from build123d import *

# Parameters (mm, degrees)
SKETCH1_W           = 72.771
SKETCH1_H           = 66.9925
SKETCH1_R           = 19.1135
SKETCH1_R_2         = 3.175
BOSS_EXTRUDE1_DEPTH = 3.175
FILLET1_R           = 2.54
SKETCH2_W           = 66.9925
SKETCH2_H           = 50.8
BOSS_EXTRUDE2_DEPTH = 3.175
BOSS_EXTRUDE5_DEPTH = 3.175
BOSS_EXTRUDE6_DEPTH = 3.175
SKETCH9_R           = 3.175
CUT_EXTRUDE1_DEPTH  = 3.175
BOSS_EXTRUDE7_DEPTH = 5.08


with BuildPart() as part:
    # Sketch1 → Boss-Extrude1 (new body)
    with BuildSketch(Plane(origin=(0, 0, 0), x_dir=(1, 0, 0), z_dir=(0, 1, 0))):
        with Locations((-3.302, 0.79375)):
            Rectangle(SKETCH1_W, SKETCH1_H)
        with Locations(Location((0, 0, 0), (0, 0, 270))):
            Circle(SKETCH1_R, mode=Mode.SUBTRACT)
        with Locations(Location((-23.5585, 23.5585, 0), (0, 0, 270))):
            Circle(SKETCH1_R_2, mode=Mode.SUBTRACT)
        with Locations(Location((23.5585, 23.5585, 0), (0, 0, 270))):
            Circle(SKETCH1_R_2, mode=Mode.SUBTRACT)
        with Locations(Location((23.5585, -23.5585, 0), (0, 0, 270))):
            Circle(SKETCH1_R_2, mode=Mode.SUBTRACT)
        with Locations(Location((-23.5585, -23.5585, 0), (0, 0, 270))):
            Circle(SKETCH1_R_2, mode=Mode.SUBTRACT)
    extrude(amount=BOSS_EXTRUDE1_DEPTH)

    # Fillet1
    fillet1_edges = [part.edges().sort_by_distance(p)[0] for p in [
        (33.0835, 1.5875, -34.29),
        (33.0835, 1.5875, 32.7025),
    ]]
    fillet(fillet1_edges, radius=FILLET1_R)

    # Sketch2 → Boss-Extrude2 (add)
    with BuildSketch(Plane.ZY.offset(39.6875)):
        with Locations((-0.79375, -25.4)):
            Rectangle(SKETCH2_W, SKETCH2_H)
    extrude(amount=-BOSS_EXTRUDE2_DEPTH)

    # Sketch7 → Boss-Extrude5 (add)
    with BuildSketch(Plane.XY.offset(32.7025)):
        Polygon((-36.5125, -50.8), (30.5435, 0), (-36.5125, 0), align=None)
    extrude(amount=-BOSS_EXTRUDE5_DEPTH)

    # Sketch8 → Boss-Extrude6 (add)
    with BuildSketch(Plane(origin=(0, 0, -34.29), x_dir=(-1, 0, 0), z_dir=(0, 0, -1))):
        Polygon((-30.5435, 0), (36.5125, 0), (36.5125, -50.8), align=None)
    extrude(amount=-BOSS_EXTRUDE6_DEPTH)

    # Sketch9 → Cut-Extrude1 (cut)
    with BuildSketch(Plane(origin=(-36.5125, 0, 0), x_dir=(0, 0, -1), z_dir=(1, 0, 0))):
        with BuildLine():
            ThreePointArc((-2.2225, -12.7), (-5.3975, -9.525), (-2.2225, -6.35))
            Line((-2.2225, -6.35), (-12.3825, -6.35))
            ThreePointArc((-12.3825, -6.35), (-10.13743597, -7.27993597), (-9.2075, -9.525))
            ThreePointArc((-9.2075, -9.525), (-10.13743597, -11.77006403), (-12.3825, -12.7))
            Line((-12.3825, -12.7), (-2.2225, -12.7))
        make_face()
        with Locations((-2.2225, -9.525)):
            Circle(SKETCH9_R)
        with Locations((-12.3825, -9.525)):
            Circle(SKETCH9_R)
        with BuildLine():
            ThreePointArc((23.8125, -12.7), (20.6375, -9.525), (23.8125, -6.35))
            Line((23.8125, -6.35), (13.6525, -6.35))
            ThreePointArc((13.6525, -6.35), (15.89756403, -7.27993597), (16.8275, -9.525))
            ThreePointArc((16.8275, -9.525), (15.89756403, -11.77006403), (13.6525, -12.7))
            Line((13.6525, -12.7), (23.8125, -12.7))
        make_face()
        with Locations((13.6525, -9.525)):
            Circle(SKETCH9_R)
        with Locations((23.8125, -9.525)):
            Circle(SKETCH9_R)
        with Locations((23.8125, -34.925)):
            Circle(SKETCH9_R)
        with BuildLine():
            Line((13.6525, -38.1), (23.8125, -38.1))
            ThreePointArc((23.8125, -38.1), (20.6375, -34.925), (23.8125, -31.75))
            Line((23.8125, -31.75), (13.6525, -31.75))
            ThreePointArc((13.6525, -31.75), (15.89756403, -32.67993597), (16.8275, -34.925))
            ThreePointArc((16.8275, -34.925), (15.89756403, -37.17006403), (13.6525, -38.1))
        make_face()
        with Locations((13.6525, -34.925)):
            Circle(SKETCH9_R)
        with Locations((-2.2225, -34.925)):
            Circle(SKETCH9_R)
        with BuildLine():
            ThreePointArc((-2.2225, -38.1), (-5.3975, -34.925), (-2.2225, -31.75))
            Line((-2.2225, -31.75), (-12.3825, -31.75))
            ThreePointArc((-12.3825, -31.75), (-10.13743597, -32.67993597), (-9.2075, -34.925))
            ThreePointArc((-9.2075, -34.925), (-10.13743597, -37.17006403), (-12.3825, -38.1))
            Line((-12.3825, -38.1), (-2.2225, -38.1))
        make_face()
        with Locations((-12.3825, -34.925)):
            Circle(SKETCH9_R)
    extrude(amount=-CUT_EXTRUDE1_DEPTH, mode=Mode.SUBTRACT)

    # Sketch10 → Boss-Extrude7 (add)
    with BuildSketch(Plane(origin=(-36.5125, 0, 0), x_dir=(0, 0, -1), z_dir=(1, 0, 0))):
        Polygon((23.8125, -15.113), (-29.5275, -15.113), (-29.5275, -29.337), (23.8125, -29.337), (31.115, -29.337), (31.115, -15.113), align=None)
        Polygon((31.115, 0), (-29.5275, 0), (-29.5275, -3.937), (23.8125, -3.937), (31.115, -3.937), align=None)
        Polygon((23.8125, -40.513), (-29.5275, -40.513), (-29.5275, -50.8), (31.115, -50.8), (31.115, -40.513), align=None)
    extrude(amount=BOSS_EXTRUDE7_DEPTH)


solid = part.part
Read the model definition and answer for the solid it produces. Units are mm, in the model's axes. A direction names the side the tool comes from. Give positions to 0.01 mm unless a question says otherwise; leave off trailing zeros. Write each loop counter-clockwise with the first axis right and the second up, starting at its lowest first coordinate (ties: lowest second). Pieces come first, ordered by that corner, then holes. Notation, with made-up numbers: (15.25, -12) -> (20.25, -12) arc R25 ccw to (20.25, 12) -> close; hole circle Ø5 at (17.5, -21.5). An arc over 180 degrees is marked (long way). Answer as a JSON object with one key per item and string values. Group by question number.
1) Consider L1, parallel to Y at x = -34, z = -6.5 (3 decimals); L2, parallel to Z at x = -31, y = -23 (1 decimal); L3, parallel to Y at x = -28, z = 23 (3 decimals). Determine where each line is inside the solid, lowest interval first. Write a range as from..to.
2) Each of these flat-tipped pins is pushed along its axis until it touches: P1, Ø1.9, axis at x = -34.5, y = -49.5, coming from the +Z side; P2, Ø10, axis at y = -42, z = -18.5, coming from the +X side; P3, Ø7.5, axis at x = 23.56, z = -23.56, coming from the -Y side. Where does it stop, or does it pass through?
3) Find section C-C (x = 0). Write down the section's boundary in (y, z) (1 decimal), and give its area (3 significant figures).
4) A tool of negligible diameter and unlimited length cuts with its end or side. For faces 4 (the flat face through (-13, -17, -34.29)), 5 (the cylindrical face through (16.1, 1.6, 10.3)), 6 (the flat face through (-14, 0, 14)), 7 (the flat face through (-34, -3.937, 0)), 8 (the cylindrical face through (-38.08, -34.99, -0.95)), from which of +Z, -Z, +X, -X, +Y, -Y can it reach the whole face along a straight path? Write none if from no direction.
5) Find section D-D (z = -16.5). Count the separate pieces of the cut face and the enclosed holes in it, and give its area (3 significant figures).
6) Find section A-A (x = 21.5). Write down the section's boundary in (y, z) (1 decimal).
7) Find section B-B (z = 24). Write down the section's boundary in (x, y) (1 decimal).
8) The mould has two halves that part along X. Classify faces 1 (the flat face through (-34, -15.113, -1)), 2 (the cylindrical face through (-22.605, 1.565, 26.587)), 3 (the flat face through (-31.433, -22, 0)): +X half, -X half, draft (parallel to the pull), parting line (faces both ways), or undercut.
Values follow:
{
 "1": {"L1": "y = -50.8..-40.513, -29.337..-15.113, -3.937..3.175", "L2": "z = -34.3..-31.1, 29.5..32.7", "L3": "y = 0..3.175"},
 "2": {"P1": "stops at z = 32.7", "P2": "stops at x = -31.43", "P3": "stops at y = 0"},
 "3": {"outline": "(-23.1, -34.3) -> (3.2, -34.3) -> (3.2, -19.1) -> (0, -19.1) -> (0, -31.1) -> (-23.1, -31.1) -> close; (-23.1, 29.5) -> (0, 29.5) -> (0, 19.1) -> (3.2, 19.1) -> (3.2, 32.7) -> (-23.1, 32.7) -> close", "area": "238 mm2"},
 "4": {"face 4": "-Z, +X, -X, +Y, -Y", "face 5": "+Y, -Y", "face 6": "+X, -Y", "face 7": "+X", "face 8": "+X, -X"},
 "5": {"separate pieces": "4", "enclosed holes": "0", "area": "435 mm2"},
 "6": {"outline": "(-6.9, -34.3) -> (3.2, -34.3) -> (3.2, -26) -> (0, -26) -> (0, -31.1) -> (-6.9, -31.1) -> close; (-6.9, 29.5) -> (0, 29.5) -> (0, 26) -> (3.2, 26) -> (3.2, 32.7) -> (-6.9, 32.7) -> close; (0, -21.1) -> (3.2, -21.1) -> (3.2, 21.1) -> (0, 21.1) -> close"},
 "7": {"outline": "(-39.7, -50.8) -> (-31.4, -50.8) -> (-31.4, -40.5) -> (-36.5, -40.5) -> (-36.5, -29.3) -> (-31.4, -29.3) -> (-31.4, -15.1) -> (-36.5, -15.1) -> (-36.5, -3.9) -> (-31.4, -3.9) -> (-31.4, 0) -> (-26.7, 0) -> (-26.7, 3.2) -> (-39.7, 3.2) -> close; (-20.4, 0) -> (20.4, 0) -> (20.4, 3.2) -> (-20.4, 3.2) -> close; (26.7, 0) -> (33.1, 0) -> (33.1, 3.2) -> (26.7, 3.2) -> close"},
 "8": {"face 1": "draft", "face 2": "undercut", "face 3": "+X half"}
}
